Job drawing, mm, ordinate dimensions from the low corner. One solid piece. A direction names the side the tool comes from. Coordinates: 2 decimals unless noted, no trailing zeros. Loops run counter-clockwise (first coordinate to the right, second up) from the corner with the lowest first, then second, coordinate; pieces in that order, holes last. Notation, with made-up numbers: (4.5, 64) -> (32.5, 64) arc R20 cw to (32.5, 99) -> close; hole circle Ø2 at (39, 59). An arc over 180 degrees is marked (long way). Use one line per item in the form item = value. Start each with the question number.
(1) Band-saw the part on B-B on z = 20.25. Give the cut face in (x, y), then the cut area to 3 significant figures.
(2) Drill centre lines: L1, parallel to X at y = 20.5, z = 18.25; L2, parallel to X at y = 43.1, z = 12.5; L3, parallel to X at y = 44.15, z = 12.5. Where is each one in solid material? Low to high. Write a range as [from, to].
(3) Mould opens along X. For the marked faces 1, 2 and 3 say: +X half, -X half, draft (parallel to the pull), parting line (faces both ways), or undercut.
(4) Band-saw the part on C-C on y = 28.5. Give the cut face in (x, z).
(5) Band-saw the part on A-A on x = 35. Give the cut face in (y, z).
(6) 3-axis set-ups, long thin cutter, end or side, ignore diameter. For the marked faces 4 and 5: which of +Z, -Z, +X, -X, +Y, -Y reach the whole face in a straight line?
(7) Band-saw the part on D-D on y = 19.5. Give the cut face in (x, z).
(8) Pin check, flat tip, straight feed: P1, Ø12.5, axis at x = 28, z = 18.5, coming from the -Y side. Stop position of the tip, or through.
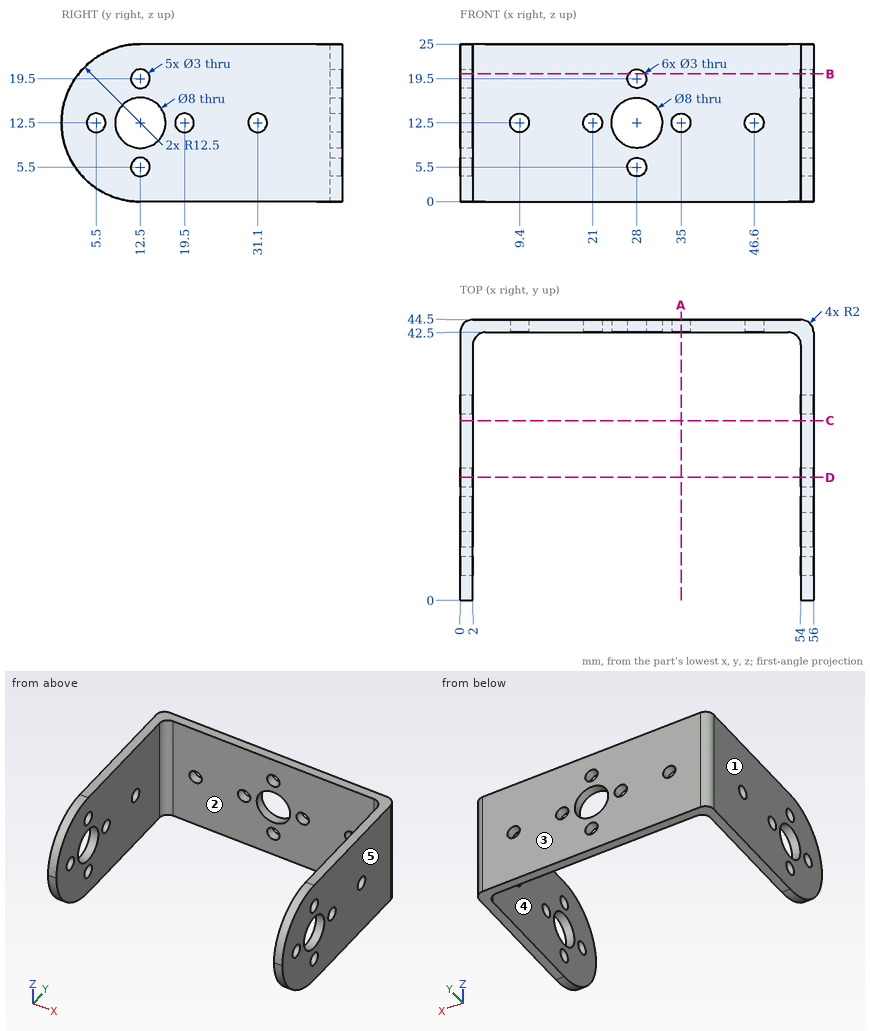
A:
q1.outline = (0, 2.69) -> (2, 2.69) -> (2, 11.2) -> (0, 11.2) -> close; (0, 13.8) -> (2, 13.8) -> (2, 40.5) arc R2 cw to (4, 42.5) -> (26.7, 42.5) -> (26.7, 44.5) -> (2, 44.5) arc R2 ccw to (0, 42.5) -> close; (29.3, 42.5) -> (52, 42.5) arc R2 cw to (54, 40.5) -> (54, 13.8) -> (56, 13.8) -> (56, 42.5) arc R2 ccw to (54, 44.5) -> (29.3, 44.5) -> close; (54, 2.69) -> (56, 2.69) -> (56, 11.2) -> (54, 11.2) -> close
q1.area = 256 mm²
q2.L1 = [0, 2], [54, 56]
q2.L2 = [0.09, 7.9], [10.9, 19.5], [22.5, 24], [32, 33.5], [36.5, 45.1], [48.1, 55.91]
q2.L3 = [0.87, 7.9], [10.9, 19.5], [22.5, 24], [32, 33.5], [36.5, 45.1], [48.1, 55.13]
q3.face_1 = -X half
q3.face_2 = undercut
q3.face_3 = draft
q4.outline = (0, 0) -> (2, 0) -> (2, 25) -> (0, 25) -> close; (54, 0) -> (56, 0) -> (56, 25) -> (54, 25) -> close
q5.outline = (42.5, 0) -> (44.5, 0) -> (44.5, 11) -> (42.5, 11) -> close; (42.5, 14) -> (44.5, 14) -> (44.5, 25) -> (42.5, 25) -> close
q6.face_4 = +Z, -Z, -Y
q6.face_5 = +Z, -Z, +X, +Y, -Y
q7.outline = (0, 0) -> (2, 0) -> (2, 11) -> (0, 11) -> close; (0, 14) -> (2, 14) -> (2, 25) -> (0, 25) -> close; (54, 0) -> (56, 0) -> (56, 11) -> (54, 11) -> close; (54, 14) -> (56, 14) -> (56, 25) -> (54, 25) -> close
q8.P1 = 42.5
